from build123d import *

# Parameters (mm, degrees)
F2_SIZE  = 0.5
F3_R     = 2
F4_DEPTH = 25


with BuildPart() as f1:
    # F0 (on Front) → F1 (revolve)
    with BuildSketch(Plane.XZ):
        Polygon((18, 0), (4, 0), (4, -20), (10, -20), (10, -8), (18, -8), align=None)
    revolve(axis=Axis((0, 0, -14.821168), (0, 0, -1)))

    # F2
    f2_edges = [f1.edges().sort_by_distance(p)[0] for p in [
        (-18, 0, 0),
        (-18, 0, -8),
        (-10, 0, -20),
        (-4, 0, 0),
        (-4, 0, -20),
    ]]
    chamfer(f2_edges, length=F2_SIZE)

    # F3 (on face) → F4 (cut)
    with BuildSketch(Plane.XY):
        with Locations((14, 0)):
            Circle(F3_R)
        with Locations((-14, 0)):
            Circle(F3_R)
        with Locations((0, 14)):
            Circle(F3_R)
        with Locations((0, -14)):
            Circle(F3_R)
    extrude(amount=-F4_DEPTH, mode=Mode.SUBTRACT)


solid = f1.part
Geometry check sheet. Reference: the model listing, model coordinates, mm. A direction names the side the tool comes from. Round coordinates to 2 decimals unless told otherwise and drop trailing zeros. Order: outer loops, then holes, each group sorted by start corner. A loop starts at its lowest first (then second) coordinate and runs counter-clockwise, first axis right, second up. Notation, with made-up numbers: M 75.5,-10.5 L 91.5,-10.5 A33 cw 91.5,27.5 Z; hole C 6,-30 d7. An arc over 180 degrees is marked long. Answer in a Markdown table with one row per item. Add a question column.
Item 1: Set-up check for faces 4 (the face through (-8, 8, -8)), 5 (the face through (4, 4, 0)): record each of +Z, -Z, +X, -X, +Y, -Y from which the full face is reachable in a straight line by a thin tool's end or side.
Item 2: Sectioned sample at A-A, the plane x = 0. State how many separate pieces and enclosed holes the cut face has, plus the area to 3 significant figures.
Item 3: Material ranges on L1, parallel to Y at x = 0, z = -6; L2, parallel to Y at x = 0, z = -10.25, recorded low to high. Write a range as [from, to].
Item 4: Depth check by flat-ended pin: pin 1 Ø6 at (x, z) = (7.5, -17.5) entering from -Y; pin 2 Ø3 at (x, y) = (-14, 0) entering from -Z; pin 3 Ø4 at (y, z) = (-11, -3) entering from +X; pin 4 Ø5 at (x, y) = (0, 14) entering from -Z. Enter the tip coordinate at first touch or a pass-through.
Item 5: Draft check along Y on faces 1 (the face through (-2.343, -17.847, -3.951)), 2 (the face through (-4.1, -2.2, -20)), 3 (the face through (0, -12, -4)). Enter one of: released by +Y, released by -Y, zero draft, split by the parting line, or undercut.
Item 6: Sectioned sample at C-C, the plane z = -15.25. Enter the section's corners in (x, y).
Filled in:
| question | item | result |
|---|---|---|
| 1 | face 4 | -Z |
| 1 | face 5 | +Z, +X, -X, +Y, -Y |
| 2 | separate pieces | 4 |
| 2 | enclosed holes | 0 |
| 2 | area | 303 mm² |
| 3 | L1 | y = [-18, -16], [-12, -4], [4, 12], [16, 18] |
| 3 | L2 | y = [-10, -4], [4, 10] |
| 4 | pin 1 | stops at y = -8.93 |
| 4 | pin 2 | passes through |
| 4 | pin 3 | stops at x = 15.59 |
| 4 | pin 4 | stops at z = -8 |
| 5 | face 1 | split by the parting line |
| 5 | face 2 | zero draft |
| 5 | face 3 | undercut |
| 6 | outline | C 0,0 d20; hole C 0,0 d8 |
